Design review of the part built by this model. Coordinates are the model's own, in mm. A direction names the side the tool comes from. Coordinates: 2 decimals unless noted, no trailing zeros. Write each loop counter-clockwise with the first axis right and the second up, starting at its lowest first coordinate (ties: lowest second). Pieces come first, ordered by that corner, then holes. Notation, with made-up numbers: M 78.25,52.25 L 137.25,52.25 A14 cw 137.25,58.25 Z; hole C 13.25,83.5 d3. An arc over 180 degrees is marked long. One line per question, with ' | ' between items.
from build123d import *

# Parameters (mm, degrees)
F1_DEPTH = 18
F2_R     = 9.2
F4_D     = 10
F5_R     = 33.5
F6_R     = 17
F7_D     = 15


with BuildPart() as f1:
    # F0 (on Right) → F1 (new body)
    with BuildSketch(Plane.YZ):
        with BuildLine():
            Line((74.743822, 13.714945), (0, 13.714945))
            Line((0, 13.714945), (-77.461272, 49.427156))
            ThreePointArc((-77.461272, 49.427156), (-85.257986, 37.247191), (-77.461272, 25.067225))
            Line((-77.461272, 25.067225), (0, -10.644986))
            Line((0, -10.644986), (74.743822, -10.644986))
            ThreePointArc((74.743822, -10.644986), (86.923788, 1.534979), (74.743822, 13.714945))
        make_face()
    extrude(amount=-F1_DEPTH)

    # F2
    f2_edges = [f1.edges().sort_by_distance(p)[0] for p in [
        (-9, -77.461272, 49.427156),
    ]]
    fillet(f2_edges, radius=F2_R)

    # F4 (through all)
    with Locations(Plane.YZ):
        with Locations((-57.928775, 26.669696), (-38.470201, 17.741643), (-24.047961, 11.102834)):
            Hole(F4_D / 2)

    # F5
    f5_edges = [f1.edges().sort_by_distance(p)[0] for p in [
        (-9, 0, -10.644986),
    ]]
    fillet(f5_edges, radius=F5_R)

    # F6
    f6_edges = [f1.edges().sort_by_distance(p)[0] for p in [
        (-9, 0, 13.714945),
    ]]
    fillet(f6_edges, radius=F6_R)

    # F7 (through all)
    with Locations(Plane.YZ):
        with Locations((25.170794, 0), (74.743822, 1.534979)):
            Hole(F7_D / 2)


solid = f1.part
1. To check wall thickness, follow line 1 along Y through (x, z) = (-11, -5); line 2 along Z through (x, y) = (-4.75, -34); line 3 along Z through (x, y) = (-16, 76.5). State the ranges of each line that lie inside material, in increasing order. Write a range as [from, to].
Answer sheet:
line 1: [-12.24, 19.58], [30.76, 71.06], [78.42, 85.02] | line 2: [5.03, 15.5], [19.98, 29.39] | line 3: [-10.52, -5.76], [8.83, 13.59]
2. Take a section at C-C (z = 0). Write out the cut boundary in (x, y), then the cut area to 3 significant figures.
Answer sheet:
outline: M -18,-23.09 L 0,-23.09 L 0,17.67 L -18,17.67 Z; M -18,32.67 L 0,32.67 L 0,67.4 L -18,67.4 Z; M -18,82.09 L 0,82.09 L 0,86.83 L -18,86.83 Z | area: 1,440 mm^2
3. Take a section at B-B (x = -9). Write out the cut boundary in (y, z), then the cut area to 3 significant figures.
Answer sheet:
outline: M -84.6,41.41 A13.41 ccw -77.46,25.07 L -6.68,-7.57 A33.5 ccw 7.35,-10.64 L 74.74,-10.64 A12.18 ccw 74.74,13.71 L 3.73,13.71 A17 cw -3.39,15.28 L -72,46.91 A9.2 ccw Z; hole C -57.93,26.67 d10; hole C -38.47,17.74 d10; hole C -24.05,11.1 d10; hole C 25.17,0 d15; hole C 74.74,1.53 d15 | area: 3,480 mm^2
4. Draft analysis for pull direction Z (two halves, no side actions). For faces 3 (the face through (-9, 41, -10.645)), 4 (the face through (-9.13, 0.04, 14.12)), 5 (the face through (-9.126, 82.237, 1.865)), state which applies: pulls with the +Z half, pulls with the -Z half, needs draft (parallel to the pull), parting line crosses it, or undercut.
Answer sheet:
face 3: pulls with the -Z half | face 4: pulls with the +Z half | face 5: undercut
5. Take a section at A-A (y = -60). Write out the cut boundary in (x, z).
Answer sheet:
outline: M -18,17.02 L 0,17.02 L 0,22.12 L -18,22.12 Z; M -18,31.22 L 0,31.22 L 0,41.38 L -18,41.38 Z
6. Tool access review of faces 1 (the face through (-9, 40, 13.715)), 2 (the face through (-8.874, -84.191, 32.005)): name each direction out of +Z, -Z, +X, -X, +Y, -Y from which nothing blocks a thin tool from reaching the whole face with its end or side.
Answer sheet:
face 1: +Z, +X, -X, +Y | face 2: +X, -X, -Y
7. Insertion check: pin 1 Ø5 at (x, z) = (-8, -4) entering from +Y; pin 2 Ø5.5 at (x, y) = (-7.5, 25.5) entering from +Z; pin 3 Ø4 at (x, z) = (-9.5, 4) entering from +Y; pin 4 Ø12 at (y, z) = (25.17, 0) entering from +X. Each pin has a flat end and moves straight along its axis. Give the tip position at first contact, or say it passes through.
Answer sheet:
pin 1: y = 86.54 | pin 2: z = 13.71 | pin 3: y = 86.91 | pin 4: through
8. Take a section at D-D (z = 20). Write out the cut boundary in (x, y), then the cut area to 3 significant figures.
Answer sheet:
outline: M -18,-66.47 L 0,-66.47 L 0,-42.93 L -18,-42.93 Z; M -18,-34.01 L 0,-34.01 L 0,-13.63 L -18,-13.63 Z | area: 790 mm^2
